For this review, take the finished solid that the model builds, in its own axes (mm). A direction names the side the tool comes from. Give positions to 0.01 mm unless a question says otherwise; leave off trailing zeros. Loops run counter-clockwise (first coordinate to the right, second up) from the corner with the lowest first, then second, coordinate; pieces in that order, holes last. Notation, with made-up numbers: (-29.5, -31.5) - (17.5, -31.5) arc R35 ccw to (17.5, 2.5) - close; hole circle Ø4 at (37.5, 44.25). An arc over 180 degrees is marked (long way). Use CSV: the item, a comma, the result in double quotes. Start each with the question number.
1. Take a section at D-D on x = 13. Give the boundary of the cut face in (y, z).
2. Take a section at A-A on y = 15. Give the boundary of the cut face in (x, z).
3. For pin 1 (8 mm diameter, centred on y = 13, z = 22.5, fed in from -X); pin 2 (8 mm diameter, centred on y = 9, z = 20, fed in from +X); pin 3 (4 mm diameter, centred on x = 0, y = 5, fed in from +Z), all flat-tipped, find the tip position at first contact; note any pin that passes through.
4. Take a section at C-C on z = 19. Give the boundary of the cut face in (x, y).
5. Mouldability with a two-part tool opening along X and no side actions: class faces 6 (the flat face through (19.566, 10, 14)), 7 (the cylindrical face through (-31.004, 5.451, 13.961)), 8 (the flat face through (-27.684, 10, 20)) as pulls with the +X half, pulls with the -X half, needs draft (parallel to the pull), parting line crosses it, or undercut.
6. Wall thickness on line 1 (X direction, y = 4.25, z = -1.5); line 2 (Z direction, x = -27, y = 13.25); line 3 (Z direction, x = -29.5, y = 4): over which ranges is each line inside the solid? List them lowest first.
7. Take a section at B-B on y = 10. Give the boundary of the cut face in (x, z), plus the area to 3 significant figures.
8. For faces 1 (the flat face through (-31, 10, 15.44)), 2 (the cylindrical face through (18.496, 5.451, 13.961)), 3 (the flat face through (-27.684, 10, -1)), 4 (the cylindrical face through (-0.065, 8.175, 28.591)), 5 (the flat face through (12.316, 10, 20)), list the 3-axis set-ups (+Z, -Z, +X, -X, +Y, -Y) from which the entire face can be reached by the end or side of a thin tool; tool diameter is ignored.
```python
from build123d import *

# Parameters (mm, degrees)
SKETCH1_W           = 40
SKETCH1_H           = 40.4
BOSS_EXTRUDE1_DEPTH = 20
SKETCH3_W           = 3
SKETCH3_H           = 20
BOSS_EXTRUDE2_DEPTH = 7.25
SKETCH5_R           = 1.5
CUT_EXTRUDE1_DEPTH  = 7.25
SKETCH6_R           = 3
BOSS_EXTRUDE3_DEPTH = 7


with BuildPart() as part:
    # Sketch1 → Boss-Extrude1 (new body)
    with BuildSketch(Plane(origin=(0, 0, 0), x_dir=(1, 0, 0), z_dir=(0, 1, 0))):
        with Locations((-7.684478372, -4.939949109)):
            Rectangle(SKETCH1_W, SKETCH1_H)
    extrude(amount=BOSS_EXTRUDE1_DEPTH)

    # Sketch3 → Boss-Extrude2 (add)
    with BuildSketch(Plane(origin=(12.315521628, 0, 0), x_dir=(0, 0, -1), z_dir=(1, 0, 0))):
        with Locations((-13.939949109, 10)):
            Rectangle(SKETCH3_W, SKETCH3_H)
    boss_extrude2 = extrude(amount=BOSS_EXTRUDE2_DEPTH)

    # Mirror1: Boss-Extrude2 across plane
    add(boss_extrude2.mirror(Plane.ZY.offset(7.684478372)))

    # Sketch5 → Cut-Extrude1 (cut)
    with BuildSketch(Plane.XY.offset(15.439949109)):
        with Locations((17.065521628, 15)):
            Circle(SKETCH5_R)
        with Locations((17.065521628, 5)):
            Circle(SKETCH5_R)
        with Locations((-32.434478372, 15)):
            Circle(SKETCH5_R)
        with Locations((-32.434478372, 5)):
            Circle(SKETCH5_R)
    extrude(amount=-CUT_EXTRUDE1_DEPTH, mode=Mode.SUBTRACT)

    # Sketch6 → Boss-Extrude3 (add)
    with BuildSketch(Plane.XY.offset(25.139949109)):
        with Locations((2.315521628, 10)):
            Circle(SKETCH6_R)
    extrude(amount=BOSS_EXTRUDE3_DEPTH)


solid = part.part
```
Check result:
1,outline,"(0, 12.44) - (20, 12.44) - (20, 15.44) - (0, 15.44) - close"
2,outline,"(-34.93, 12.44) - (-33.93, 12.44) - (-33.93, 15.44) - (-34.93, 15.44) - close; (-30.93, 12.44) - (-27.68, 12.44) - (-27.68, -15.26) - (12.32, -15.26) - (12.32, 12.44) - (15.57, 12.44) - (15.57, 15.44) - (12.32, 15.44) - (12.32, 25.14) - (-27.68, 25.14) - (-27.68, 15.44) - (-30.93, 15.44) - close; (18.57, 12.44) - (19.57, 12.44) - (19.57, 15.44) - (18.57, 15.44) - close"
3,pin 1,"stops at x = -27.68"
3,pin 2,"stops at x = 12.32"
3,pin 3,"stops at z = 25.14"
4,outline,"(-27.68, 0) - (12.32, 0) - (12.32, 20) - (-27.68, 20) - close"
5,face 6,"pulls with the +X half"
5,face 7,"undercut"
5,face 8,"pulls with the -X half"
6,line 1,"x = -27.68 to 12.32"
6,line 2,"z = -15.26 to 25.14"
6,line 3,"z = 12.44 to 15.44"
7,outline,"(-34.93, 12.44) - (-27.68, 12.44) - (-27.68, -15.26) - (12.32, -15.26) - (12.32, 12.44) - (19.57, 12.44) - (19.57, 15.44) - (12.32, 15.44) - (12.32, 25.14) - (5.32, 25.14) - (5.32, 32.14) - (-0.68, 32.14) - (-0.68, 25.14) - (-27.68, 25.14) - (-27.68, 15.44) - (-34.93, 15.44) - close"
7,area,"1,700 mm²"
8,face 1,"+Z, -X, +Y, -Y"
8,face 2,"+Z, -Z"
8,face 3,"-Z, -X, +Y, -Y"
8,face 4,"+Z"
8,face 5,"+Z, +X, +Y, -Y"
